Could you check a few things on this model? Use its own coordinates, in mm. Coordinates: 2 decimals unless noted, no trailing zeros. Write each loop counter-clockwise with the first axis right and the second up, starting at its lowest first coordinate (ties: lowest second). Pieces come first, ordered by that corner, then holes.
Item 1: If I drill on probe 1 along Z at (x, y) = (12.7, 0.95); probe 2 along Z at (x, y) = (0, 1.15); probe 3 along Z at (x, y) = (25.4, 0.3), over which ranges is the centre line in solid material (lowest first)?
Item 2: I want a section at C-C on x = -22. Please give me the cut outline in (y, z), then the cut area to 3 significant figures.
Item 3: I want a section at B-B on z = -45.5. Please give me the cut outline in (x, y), then the cut area to 3 significant figures.
Item 4: I want a section at A-A on y = 0.75. State how many separate pieces and enclosed holes the cut face has, then the cut area to 3 significant figures.
Item 5: For P1, Ø0.5, axis at y = 0.5, z = -20, coming from the +X side, with a flat end and sliding along its axis, tell me the tip position at first contact or that it passes through.
Autodesk Inventor part; units mm, degrees
ref_plane "YZ Plane" through (0, 0, 0) normal (1, 0, 0) x (0, 1, 0)
ref_plane "XZ Plane" through (0, 0, 0) normal (0, 1, 0) x (-1, 0, 0)
ref_plane "XY Plane" through (0, 0, 0) normal (0, 0, 1) x (1, 0, 0)
sketch "main" plane through (0, 0, 0) normal (0, 0, 1) x (1, 0, 0)
  arc A0 (-6.1043, -28.9805) -> (-0.9888, -26.4406) centre (-6.0688, -22.6306) ccw
  arc A1 (-31.4687, -16.2806) -> (-31.4687, -28.9806) centre (-31.4688, -22.6306) ccw
  circle A2 centre (-6.0688, -22.6306) radius 2.0955
  circle A3 centre (-31.4688, -22.6306) radius 2.0955
  line L0 (-10.8313, -16.2806) -> (-31.4688, -16.2806)
  line L1 (-6.0331, -28.9805) -> (-31.4687, -28.9806)
  circle A4 centre (-6.0688, 28.169) radius 2.0955
  circle A5 centre (6.6312, 28.1694) radius 2.0955
  line L2 (0.2812, 15.4694) -> (0.2812, -2.5222)
  line L3 (37.1112, 24.3594) -> (-0.9888, -26.4406)
  line L4 (-18.7688, 21.8194) -> (-6.0688, 21.8194)
  arc A6 (0.2812, 15.4694) -> (-6.0688, 21.8194) centre (-6.0688, 15.4694) ccw
  arc A7 (-18.6975, 34.519) -> (-18.7688, 21.8194) centre (-18.7688, 28.1694) ccw
  line L5 (-18.6975, 34.519) -> (6.6312, 34.519)
  circle A8 centre (32.0312, 28.1694) radius 2.0955
  arc A9 (37.1112, 24.3594) -> (32.0311, 34.5194) centre (32.0312, 28.1694) ccw
  line L6 (6.6311, 34.519) -> (32.0311, 34.5194)
  circle A10 centre (-18.7688, 28.1694) radius 2.0956
  line L7 (-0.3538, -4.4272) -> (-8.2913, -15.0106)
  arc A11 (-10.8313, -16.2806) -> (-8.2913, -15.0106) centre (-10.8313, -13.1056) ccw
  arc A12 (-0.3538, -4.4272) -> (0.2812, -2.5222) centre (-2.8938, -2.5222) ccw
  point P0 (-4.0049, 2.2465)
  point P1 (0.2812, -3.5806)
  dimension "d0" = 4.191
  dimension "d1" = 4.191
  dimension "d2" = 12.7
  dimension "d4" = 6.35
  dimension "d7" = 6.35
  dimension "d8" = 25.4
  dimension "d9" = 3.175
sketch "Sketch1" plane through (0, 0, 0) normal (0, 1, 0) x (-1, 0, 0)
  arc A0 (-0.0356, -57.1495) -> (5.08, -54.6096) centre (0, -50.7996) ccw
  arc A1 (-25.4, -44.4496) -> (-25.4, -57.1496) centre (-25.4, -50.7996) ccw
  circle A2 centre (0, -50.7996) radius 2.0955
  circle A3 centre (-25.4, -50.7996) radius 2.0955
  line L0 (-4.7625, -44.4496) -> (-25.4, -44.4496)
  line L1 (0.0356, -57.1495) -> (-25.4, -57.1496)
  circle A4 centre (0, 0) radius 2.0955
  circle A5 centre (12.7, 0.0004) radius 2.0955
  line L2 (6.35, -12.6996) -> (6.35, -30.6913)
  line L3 (43.18, -3.8096) -> (5.08, -54.6096)
  line L4 (-12.7, -6.3496) -> (0, -6.3496)
  arc A6 (6.35, -12.6996) -> (0, -6.3496) centre (0, -12.6996) ccw
  arc A7 (-12.6287, 6.35) -> (-12.7, -6.3496) centre (-12.7, 0.0004) ccw
  line L5 (-12.6287, 6.35) -> (12.7, 6.35)
  circle A8 centre (38.1, 0.0004) radius 2.0955
  arc A9 (43.18, -3.8096) -> (38.0999, 6.3504) centre (38.1, 0.0004) ccw
  line L6 (12.6999, 6.35) -> (38.0999, 6.3504)
  circle A10 centre (-12.7, 0.0004) radius 2.0956
  line L7 (5.715, -32.5963) -> (-2.2225, -43.1796)
  arc A11 (-4.7625, -44.4496) -> (-2.2225, -43.1796) centre (-4.7625, -41.2746) ccw
  arc A12 (5.715, -32.5963) -> (6.35, -30.6913) centre (3.175, -30.6913) ccw
  point P0 (12.7, 6.35)
  point P1 (12.7, 6.35)
extrude "Extrusion1" add sketch "Sketch1" along normal blind 1.5875
properties part number "gusset" material "Acetal Resin, White"
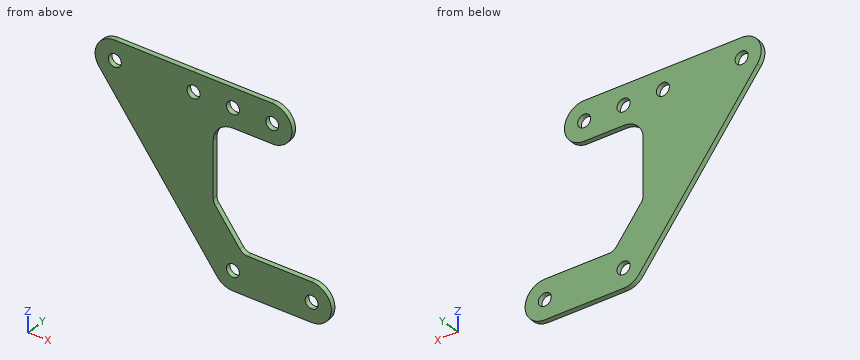
Response values:
1. probe 1: z = -57.15 to -44.45, -6.35 to -2.1, 2.1 to 6.35
1. probe 2: z = -57.15 to -52.9, -48.7 to -40.22, -6.35 to -2.1, 2.1 to 6.35
1. probe 3: z = -57.15 to -52.9, -48.7 to -44.45
2. outline: (0, -32.05) - (1.59, -32.05) - (1.59, 6.35) - (0, 6.35) - close
2. area: 61.0 mm2
3. outline: (-11.91, 0) - (28.9, 0) - (28.9, 1.59) - (-11.91, 1.59) - close
3. area: 64.8 mm2
4. separate pieces: 1
4. enclosed holes: 6
4. area: 2,030 mm2
5. P1: stops at x = -6.35
